from build123d import *

# Parameters (mm, degrees)
DODANIE_WYCI_GNI_CIE1_DEPTH = 20
SFAZOWANIE1_SIZE            = 1.267383774
SFAZOWANIE1_SIZE_2          = 1
SZKIC2_R                    = 1.75
WYTNIJ_WYCI_GNI_CIE1_DEPTH  = 10
WYTNIJ_WYCI_GNI_CIE2_START  = -1
SZKIC3_R                    = 1.75
WYTNIJ_WYCI_GNI_CIE2_DEPTH  = 1
DODANIE_WYCI_GNI_CIE2_START = -20
DODANIE_WYCI_GNI_CIE2_DEPTH = 20
SZKIC5_R                    = 3.5
WYTNIJ_WYCI_GNI_CIE3_DEPTH  = 20
ZAOKR_GLENIE1_R             = 10


with BuildPart() as part:
    # Szkic1 → Dodanie-wyciągnięcie1 (new body)
    with BuildSketch(Plane.XY):
        with BuildLine():
            ThreePointArc((5.2, 0), (-3.304542328, -4.01497198), (-1, 5.102940329))
            Line((-1, 5.102940329), (-1, 9.949874371))
            ThreePointArc((-1, 9.949874371), (-3.068514323, 9.517574263), (-5, 8.660254038))
            ThreePointArc((-5, 8.660254038), (-5, -8.660254038), (10, 0))
            ThreePointArc((10, 0), (8.660254038, 5), (5, 8.660254038))
            ThreePointArc((5, 8.660254038), (3.068514323, 9.517574263), (1, 9.949874371))
            Line((1, 9.949874371), (1, 5.102940329))
            ThreePointArc((1, 5.102940329), (4.01497198, 3.304542328), (5.2, 0))
        make_face()
        with BuildLine():
            ThreePointArc((-5, 8.660254038), (-3.068514323, 9.517574263), (-1, 9.949874371))
            Line((-1, 9.949874371), (-1, 19.949874371))
            Line((-1, 19.949874371), (-5, 19.949874371))
            Line((-5, 19.949874371), (-5, 8.660254038))
        make_face()
        with BuildLine():
            Line((1, 19.949874371), (1, 9.949874371))
            ThreePointArc((1, 9.949874371), (3.068514323, 9.517574263), (5, 8.660254038))
            Line((5, 8.660254038), (5, 19.949874371))
            Line((5, 19.949874371), (1, 19.949874371))
        make_face()
    extrude(amount=DODANIE_WYCI_GNI_CIE1_DEPTH)

    # Sfazowanie1
    # the kernel refuses this chamfer: 1.267383774, 1 mm, written as the material it takes off along each edge
    with BuildSketch(Plane(origin=(-1, 5.102940329, -3.274401996), x_dir=(0, 1, 0), z_dir=(0, 0, 1))) as sfazowanie1_piece_1:
        with BuildLine():
            Line((SFAZOWANIE1_SIZE, 0), (-0.336229117, 1.078091485))
            ThreePointArc((-0.336229117, 1.078091485), (-0.144735056, 0.567227001), (0, 0))
            Line((0, 0), (SFAZOWANIE1_SIZE, 0))
        make_face()
    extrude(amount=26.548803992, mode=Mode.SUBTRACT)
    with BuildSketch(Plane(origin=(1, 5.102940329, -4.38469538), x_dir=(0.9364406344520153, -0.35082607962793627, 0), z_dir=(0, 0, 1))) as sfazowanie1_piece_2:
        with BuildLine():
            Line((1.707607831, 0), (-SFAZOWANIE1_SIZE_2 * 0.350826079628, SFAZOWANIE1_SIZE_2 * 0.936440634452))
            Line((-SFAZOWANIE1_SIZE_2 * 0.350826079628, SFAZOWANIE1_SIZE_2 * 0.936440634452), (0, 0))
            ThreePointArc((0, 0), (0.877241421, 0.070520422), (1.707607831, 0))
        make_face()
    extrude(amount=28.76939076, mode=Mode.SUBTRACT)
    # the kernel refuses this chamfer: 1.267383774, 1 mm, written as the material it takes off along each edge
    with BuildSketch(Plane(origin=(0, 0, 20), x_dir=(0.05297189927018693, 0.9985960033405447, 0), z_dir=(0.9985960033405447, -0.05297189927018693, 0))) as sfazowanie1_2_piece_1:
        Polygon((5.2 + SFAZOWANIE1_SIZE_2, 0), (5.2, -SFAZOWANIE1_SIZE_2), (5.2, 0), align=None)
    revolve(axis=Axis((0, 0, 20), (0, 0, 1)), revolution_arc=359.64, mode=Mode.SUBTRACT)

    # Szkic2 → Wytnij-wyciągnięcie1 (cut)
    with BuildSketch(Plane(origin=(5, 0, 0), x_dir=(0, 0, -1), z_dir=(1, 0, 0))):
        with Locations((-14, 13.949874371)):
            Circle(SZKIC2_R)
        with Locations((-6, 13.949874371)):
            Circle(SZKIC2_R)
    extrude(amount=-WYTNIJ_WYCI_GNI_CIE1_DEPTH, mode=Mode.SUBTRACT)

    # Szkic3 → Wytnij-wyciągnięcie2 (cut)
    # profile 1 of 2: a face of its own
    with BuildSketch(Plane.ZY.offset(5).offset(WYTNIJ_WYCI_GNI_CIE2_START)):
        Polygon((9.464101615, 13.949874371), (7.732050808, 16.949874371), (4.267949192, 16.949874371), (2.535898385, 13.949874371), (4.267949192, 10.949874371), (7.732050808, 10.949874371), align=None)
        with Locations(Location((6, 13.949874371, 0), (0, 0, 270))):
            Circle(SZKIC3_R, mode=Mode.SUBTRACT)
    # profile 2 of 2: a face of its own
    with BuildSketch(Plane.ZY.offset(5).offset(WYTNIJ_WYCI_GNI_CIE2_START)):
        Polygon((10.535898385, 13.949874371), (12.267949192, 10.949874371), (15.732050808, 10.949874371), (17.464101615, 13.949874371), (15.732050808, 16.949874371), (12.267949192, 16.949874371), align=None)
        with Locations(Location((14, 13.949874371, 0), (0, 0, 270))):
            Circle(SZKIC3_R, mode=Mode.SUBTRACT)
    extrude(amount=WYTNIJ_WYCI_GNI_CIE2_DEPTH, mode=Mode.SUBTRACT)

    # Szkic4 → Dodanie-wyciągnięcie2 (add)
    with BuildSketch(Plane.XY.offset(20).offset(DODANIE_WYCI_GNI_CIE2_START)):
        with BuildLine():
            ThreePointArc((10, 0), (7.071067812, -7.071067812), (0, -10))
            Line((0, -10), (25, -10))
            Line((25, -10), (25, 0))
            Line((25, 0), (10, 0))
        make_face()
    extrude(amount=DODANIE_WYCI_GNI_CIE2_DEPTH)

    # Szkic5 → Wytnij-wyciągnięcie3 (cut)
    with BuildSketch(Plane(origin=(0, 0, 0), x_dir=(1, 0, 0), z_dir=(0, 1, 0))):
        with Locations(Location((17.5, -10, 0), (0, 0, 270))):
            Circle(SZKIC5_R)
    extrude(amount=-WYTNIJ_WYCI_GNI_CIE3_DEPTH, mode=Mode.SUBTRACT)

    # Zaokrąglenie1
    zaokr_glenie1_edges = [part.edges().sort_by_distance(p)[0] for p in [
        (25, -5, 20),
    ]]
    fillet(zaokr_glenie1_edges, radius=ZAOKR_GLENIE1_R)


solid = part.part
Geometry: final body of the model. Coordinates: model frame, mm. A direction names the side the tool comes from. Coordinates: 2 decimals unless noted, no trailing zeros. Write each loop counter-clockwise with the first axis right and the second up, starting at its lowest first coordinate (ties: lowest second). Pieces come first, ordered by that corner, then holes. Notation, with made-up numbers: (-25, 50.5) - (-20, 50.5) arc R25 ccw to (-20, 65.5) - close; hole circle Ø4 at (3, -27). An arc over 180 degrees is marked (long way). Return JSON: item names as keys, results as strings.
Item 1: Section query B-B (x = 17.5). Output: boundary loops of the cut face in (y, z).
Completed:
{"outline": "(-10, 0) - (0, 0) - (0, 6.5) - (-10, 6.5) - close; (-10, 13.5) - (0, 13.5) - (0, 19.68) - (-10, 19.68) - close"}
Item 2: Section query A-A (z = 6). Output: boundary loops of the cut face in (x, y), and give its area (3 significant figures).
Completed:
{"outline": "(-5, 8.66) arc R10 ccw to (0, -10) - (25, -10) - (25, 0) - (10, 0) arc R10 ccw to (5, 8.66) - (5, 12.2) - (1, 12.2) - (1, 6.1) - (2.6, 4.5) arc R5.2 cw (long way) to (-2.08, 4.77) - (-1, 6.37) - (-1, 12.2) - (-4, 12.2) - (-4, 10.95) - (-5, 10.95) - close; (-5, 16.95) - (-4, 16.95) - (-4, 15.7) - (-1, 15.7) - (-1, 19.95) - (-5, 19.95) - close; (1, 15.7) - (5, 15.7) - (5, 19.95) - (1, 19.95) - close", "area": "443 mm2"}
Item 3: Pin query (flat end, axial travel): pin 1 Ø7 at (y, z) = (15.5, 7.5) entering from -X; pin 2 Ø12 at (x, y) = (0, 0) entering from +Z; pin 3 Ø5.5 at (y, z) = (13.95, 6) entering from +X; pin 4 Ø12 at (x, y) = (8.5, -3) entering from -Z. Return the tip coordinate at first contact, or that it passes through.
Completed:
{"pin 1": "stops at x = -5", "pin 2": "stops at z = 19.8", "pin 3": "stops at x = 5", "pin 4": "stops at z = 0"}
Item 4: Reachability of faces 1 (the face through (14, 0, 8)), 2 (the face through (-4.49, 12.47, 11.39)), 3 (the face through (25, -5, 5)) from +Z, -Z, +X, -X, +Y, -Y: full face, straight path, thin tool, end or side. Return the list, or none.
Completed:
{"face 1": "+Z, -Z, +X, +Y", "face 2": "-X", "face 3": "+Z, -Z, +X, +Y, -Y"}
Item 5: Line query: L1, parallel to X at y = 11.25, z = 3; L2, parallel to Y at x = 2.3, z = 6; L3, parallel to Y at x = -2.15, z = 14. Output: solid intervals per line, ascending.
Completed:
{"L1": "x = -5 to -1, 1 to 5", "L2": "y = -10 to -4.66, 4.8 to 12.2, 15.7 to 19.95", "L3": "y = -9.77 to -4.73, 4.73 to 12.2, 15.7 to 19.95"}
Item 6: Pull-direction query (X, two-part tool) for faces 4 (the face through (-4.493, 12.429, 8.586)), 5 (the face through (1, 13, 10)), 6 (the face through (21.99, -4.93, 17.15)), 7 (the face through (-0.1, -5.4, 19.2)); classes: +X half, -X half, draft (parallel to the pull), parting line (faces both ways), or undercut.
Completed:
{"face 4": "draft", "face 5": "undercut", "face 6": "+X half", "face 7": "undercut"}
Item 7: Section query C-C (y = 13.25). Count the separate pieces of the cut face and the enclosed holes in it, and give its area (3 significant figures).
Completed:
{"separate pieces": "6", "enclosed holes": "0", "area": "103 mm2"}
